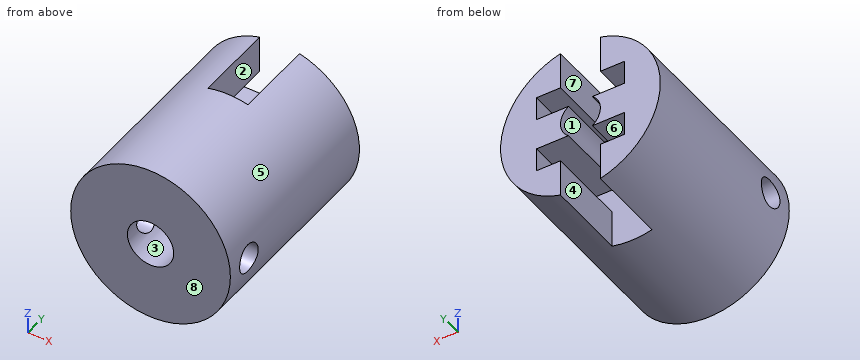
Autodesk Inventor part; units mm, degrees
ref_plane "YZ Plane" through (0, 0, 0) normal (1, 0, 0) x (0, 1, 0)
ref_plane "XZ Plane" through (0, 0, 0) normal (0, 1, 0) x (-1, 0, 0)
ref_plane "XY Plane" through (0, 0, 0) normal (0, 0, 1) x (1, 0, 0)
sketch "Sketch1" plane through (0, 0, 0) normal (0, 1, 0) x (-1, 0, 0)
  circle A0 centre (0, 0) radius 12.7
  dimension "d0" = 25.4
extrude "Extrusion1" add sketch "Sketch1" along normal blind 31.75
sketch "Sketch3" plane through (0, 31.75, 0) normal (0, 1, 0) x (1, 0, 0)
  circle A0 centre (0, 0) radius 12.7
  line L0 (0, -12.7) -> (-3.175, -12.7)
  line L1 (-3.175, -12.7) -> (-3.175, -6.35)
  line L2 (-3.175, -6.35) -> (-6.985, -6.35)
  line L3 (-6.985, -6.35) -> (-6.985, -2.54)
  line L4 (-6.985, -2.54) -> (0, -2.54)
  line L5 (0, -12.7) -> (0, -2.54)
  line L6 (0, -12.7) -> (3.175, -12.7)
  line L7 (3.175, -12.7) -> (3.175, -6.35)
  line L8 (3.175, -6.35) -> (6.985, -6.35)
  line L9 (6.985, -6.35) -> (6.985, -2.54)
  line L10 (6.985, -2.54) -> (0, -2.54)
  point P0 (-3.175, -12.2967)
  point P1 (3.175, -12.2967)
  dimension "d3" = 3.175
  dimension "d4" = 6.35
  dimension "d5" = 3.81
  dimension "d6" = 3.81
extrude "Extrusion2" cut sketch "Sketch3" against normal blind 12.7 contours L1 L2 L3 L4 L5 A0 | A0 L5 L10 L9 L8 L7
mirror "Mirror1" about plane through (0, 0, 0) normal (0, 0, 1) of "Extrusion2"
sketch "Sketch4" plane through (0, 31.75, 0) normal (0, 1, 0) x (1, 0, 0)
  point P0 (0, 0)
  point P1 (0, 0)
hole "Hole1" at (0, 31.75, 0) direction (0, -1, 0) diameter 6.35 depth 12.7
sketch "Sketch5" plane through (0, 0, 0) normal (0, -1, 0) x (1, 0, 0)
  point P0 (0, 0)
  point P1 (0, 0)
hole "Hole2" at (0, 0, 0) direction (0, 1, 0) diameter 7.366 depth 12.7
sketch "Sketch8" plane through (0, 0, 0) normal (1, 0, 0) x (0, 1, 0)
  circle A0 centre (4.572, 0) radius 2.286
  line L0 (0, -12.7) -> (0, 12.7)
  point P0 (0, 0)
  dimension "d33" = 4.572
  dimension "d34" = 4.572
extrude "Extrusion5" cut sketch "Sketch8" along normal mid plane 25.4
properties part number "hub"
Verification items for the finished model (mm, model axes). Face numbers are marked on the shaded views. A direction names the side the tool comes from. Give positions to 0.01 mm unless a question says otherwise; leave off trailing zeros. Order: outer loops, then holes, each group sorted by start corner. A loop starts at its lowest first (then second) coordinate and runs counter-clockwise, first axis right, second up. Notation, with made-up numbers: M 42.5,-30.75 L 82.5,-30.75 A14 ccw 82.5,-3.75 Z; hole C 5,-5.5 d5. An arc over 180 degrees is marked long. Answer as a JSON object with one key per item and string values. Group by question number.
1) Cross-section at A-A (y = 20). Enter the section's corners in (x, z) (3 decimals), then the cut area to 3 significant figures.
2) Access from +Z, -Z, +X, -X, +Y, -Y to the whole of each face (thin tool, end or side, straight path). Record for the marked faces 1, 2, 3 and 4.
3) Scan lines: line 1 along X through (y, z) = (9.25, 0); line 2 along X through (y, z) = (20.5, -11) (3 decimals). Record each from-to range of solid material in increasing order. Write a range as [from, to].
4) Depth check by flat-ended pin: pin 1 Ø1.5 at (y, z) = (14.5, 2.5) entering from +X; pin 2 Ø2.5 at (x, y) = (4.5, 28) entering from -Z; pin 3 Ø1.5 at (x, y) = (-3, 23.5) entering from +Z. Enter the tip coordinate at first touch or a pass-through.
5) Cross-section at D-D (y = 8.5). Enter the section's corners in (x, z), then the cut area to 3 significant figures.
6) Cross-section at C-C (x = 0). Enter the section's corners in (y, z), then the cut area to 3 significant figures.
7) Mould release check, pull along X, two halves, no side actions. Record for the marked faces 5, 6, 7 and 8: released by +X, released by -X, zero draft, split by the parting line, or undercut.
8) Cross-section at B-B (z = 0). Enter the section's corners in (x, y) (3 decimals), then the cut area to 3 significant figures.
Result sheet:
{
 "1": {"outline": "M -6.985,-6.35 L -6.985,-2.54 L -1.905,-2.54 A3.175 cw -1.905,2.54 L -6.985,2.54 L -6.985,6.35 L -3.175,6.35 L -3.175,12.297 A12.7 ccw -3.175,-12.297 L -3.175,-6.35 Z; M 1.905,-2.54 L 6.985,-2.54 L 6.985,-6.35 L 3.175,-6.35 L 3.175,-12.297 A12.7 ccw 3.175,12.297 L 3.175,6.35 L 6.985,6.35 L 6.985,2.54 L 1.905,2.54 A3.175 cw Z", "area": "293 mm2"},
 "2": {"face 1": "+Y", "face 2": "+Z, +Y", "face 3": "-Y", "face 4": "-Z, +Y"},
 "3": {"line 1": "x = [-12.7, -3.68], [3.68, 12.7]", "line 2": "x = [-6.347, -3.175], [3.175, 6.347]"},
 "4": {"pin 1": "stops at x = 12.58", "pin 2": "stops at z = -12.28", "pin 3": "stops at z = 12.3"},
 "5": {"outline": "C 0,0 d25.4; hole C 0,0 d7.37", "area": "464 mm2"},
 "6": {"outline": "M 0,-12.7 L 19.05,-12.7 L 19.05,12.7 L 0,12.7 L 0,3.68 L 12.7,3.68 L 12.7,-3.68 L 0,-3.68 Z", "area": "390 mm2"},
 "7": {"face 5": "split by the parting line", "face 6": "undercut", "face 7": "undercut", "face 8": "zero draft"},
 "8": {"outline": "M -12.7,0 L -3.683,0 L -3.683,2.286 L -12.7,2.286 Z; M -12.7,6.858 L -3.683,6.858 L -3.683,12.7 L 3.683,12.7 L 3.683,6.858 L 12.7,6.858 L 12.7,31.75 L 3.175,31.75 L 3.175,19.05 L -3.175,19.05 L -3.175,31.75 L -12.7,31.75 Z; M 3.683,0 L 12.7,0 L 12.7,2.286 L 3.683,2.286 Z", "area": "550 mm2"}
}
